```python
from build123d import *

# Parameters (mm, degrees)
ESBO_O1_R                = 1.5
RESSALTO_EXTRUS_O1_DEPTH = 2


with BuildPart() as part:
    # Esboço1 → Ressalto-extrusão1 (new body)
    with BuildSketch(Plane.XY):
        with BuildLine():
            Line((-1.121038668, 3.291347086), (0.008712569, 3.291347086))
            ThreePointArc((0.008712569, 3.291347086), (7.079780381, 0.362414898), (10.008712569, -6.708652914))
            Line((10.008712569, -6.708652914), (10.008712569, -30.785558293))
            ThreePointArc((10.008712569, -30.785558293), (9.130032913, -32.906878637), (7.008712569, -33.785558293))
            Line((7.008712569, -33.785558293), (5.878961332, -33.785558293))
            ThreePointArc((5.878961332, -33.785558293), (-1.19210648, -30.856626105), (-4.121038668, -23.785558293))
            Line((-4.121038668, -23.785558293), (-4.121038668, 0.291347086))
            ThreePointArc((-4.121038668, 0.291347086), (-3.242359012, 2.41266743), (-1.121038668, 3.291347086))
        make_face()
        Circle(ESBO_O1_R, mode=Mode.SUBTRACT)
        with Locations((5.236066432, -25.02000308)):
            Circle(ESBO_O1_R, mode=Mode.SUBTRACT)
    extrude(amount=RESSALTO_EXTRUS_O1_DEPTH)


solid = part.part
```
Check sheet for the modelled part. Datum: model origin and axes. Units: mm. Round coordinates to 2 decimals unless told otherwise and drop trailing zeros. Order: outer loops, then holes, each group sorted by start corner. A loop starts at its lowest first (then second) coordinate and runs counter-clockwise, first axis right, second up.
1) Go/stop test with a flat-tipped pin: pin 1 Ø1 at (x, z) = (8.5, 0.5) entering from -Y. Record where the tip stops, or that it passes through.
2) Section check C-C (x = 6.25). Record the boundary of the cut face in (y, z), and give its area (3 significant figures).
3) Section check B-B (x = -0.5). Record the boundary of the cut face in (y, z).
4) Mould release check, pull along Y, two halves, no side actions. Record for faces 1 (the flat face through (6.5, -33.786, 1)), 2 (the cylindrical face through (4.911, -26.484, 0.986)), 3 (the flat face through (10.009, -19, 1)), 4 (the cylindrical face through (-1.5, 0.07, 0.99)): +Y half, -Y half, draft (parallel to the pull), parting line (faces both ways), or undercut.
5) Scan lines: line 1 (Y direction, x = 6, z = 0.1); line 2 (X direction, y = -1, z = 1.35); line 3 (Y direction, x = 0, z = 1.55). Record each from-to range of solid material in increasing order.
6) Section check D-D (x = -3). Record the boundary of the cut face in (y, z), and give its area (3 significant figures).
7) Section check A-A (z = 0.5). Record the boundary of the cut face in (x, y).
Result:
1. pin 1: stops at y = -33.62
2. outline: (-33.79, 0) - (-26.13, 0) - (-26.13, 2) - (-33.79, 2) - close; (-23.91, 0) - (1.1, 0) - (1.1, 2) - (-23.91, 2) - close
2. area: 65.4 mm2
3. outline: (-31.49, 0) - (-1.41, 0) - (-1.41, 2) - (-31.49, 2) - close; (1.41, 0) - (3.29, 0) - (3.29, 2) - (1.41, 2) - close
4. face 1: -Y half
4. face 2: undercut
4. face 3: draft
4. face 4: undercut
5. line 1: y = -33.79 to -26.31, -23.73 to 1.3
5. line 2: x = -4.12 to -1.12, 1.12 to 8.22
5. line 3: y = -31.87 to -1.5, 1.5 to 3.29
6. outline: (-28.39, 0) - (2.63, 0) - (2.63, 2) - (-28.39, 2) - close
6. area: 62.0 mm2
7. outline: (-4.12, -23.79) arc R10 ccw to (5.88, -33.79) - (7.01, -33.79) arc R3 ccw to (10.01, -30.79) - (10.01, -6.71) arc R10 ccw to (0.01, 3.29) - (-1.12, 3.29) arc R3 ccw to (-4.12, 0.29) - close; hole circle Ø3 at (0, 0); hole circle Ø3 at (5.24, -25.02)
